Autodesk Inventor part; units mm, degrees
ref_plane "YZ Plane" through (0, 0, 0) normal (1, 0, 0) x (0, 1, 0)
ref_plane "XZ Plane" through (0, 0, 0) normal (0, 1, 0) x (-1, 0, 0)
ref_plane "XY Plane" through (0, 0, 0) normal (0, 0, 1) x (1, 0, 0)
sketch "Sketch1" plane through (0, 0, 0) normal (0, 1, 0) x (-1, 0, 0)
  circle A0 centre (0, 0) radius 2.5
  circle A1 centre (0, 0) radius 3.5
  dimension "d228" = 5
  dimension "d229" = 7
extrude "Extrusion1" add sketch "Sketch1" along normal blind 2
sketch "Sketch2" plane through (0, 2, 0) normal (0, 1, 0) x (1, 0, 0)
  circle A0 centre (0, 0) radius 3.5
  circle A1 centre (0, 0) radius 3.5
  line L0 (-16, -2) -> (0, -3.5)
  circle A2 centre (0, 0) radius 3.5
  line L1 (0, 3.5) -> (-16, 2)
  circle A3 centre (-14, 0) radius 0.75
  arc A4 (-16, 2) -> (-16, -2) centre (-16, 0) ccw
  circle A5 centre (0, 0) radius 1
  circle A6 centre (0, 0) radius 2.5
  circle A7 centre (0, 0) radius 2.5
  dimension "d234" = 1.5
  dimension "d236" = 16
  dimension "d237" = 2
  dimension "d238" = 2
  dimension "d241" = 2
extrude "Extrusion2" add sketch "Sketch2" along normal blind 2 contours A0 L0 L1 | A0 L0 A4 L1
extrude "Extrusion3" add sketch "Sketch2" along normal blind 1 contours A6
extrude "Extrusion4" cut sketch "Sketch2" along normal blind 0.5 contours A6
properties part number "Langbektang houder"
Geometry: final body of the model. Coordinates: model frame, mm. A direction names the side the tool comes from. Coordinates: 2 decimals unless noted, no trailing zeros. Order: outer loops, then holes, each group sorted by start corner. A loop starts at its lowest first (then second) coordinate and runs counter-clockwise, first axis right, second up. Notation, with made-up numbers: (11, 60) - (44, 60) arc R36 cw to (44, 95) - close; hole circle Ø8 at (18, -4). An arc over 180 degrees is marked (long way). Write each question's results on one line, items separated by ' | '.
(1) Section query D-D, the plane y = 0.6. Return the cut outline in (x, z).
Values found:
outline: circle Ø7 at (0, 0); hole circle Ø5 at (0, 0)
(2) Line query: line 1 (X direction, y = 2.9, z = 0); line 2 (X direction, y = 3.4, z = 0); line 3 (Z direction, x = 0, y = 1.45). Output: solid intervals per line, ascending. Write a range as [from, to].
Values found:
line 1: x = [-18, -14.75], [-13.25, -1], [1, 3.5] | line 2: x = [-18, -14.75], [-13.25, -2.5], [2.5, 3.5] | line 3: z = [-3.5, -2.5], [2.5, 3.5]
(3) Section query C-C, the plane x = -14. Return the cut outline in (y, z), plus the area to 3 significant figures.
Values found:
outline: (2, -2.19) - (4, -2.19) - (4, -0.75) - (2, -0.75) - close; (2, 0.75) - (4, 0.75) - (4, 2.19) - (2, 2.19) - close | area: 5.75 mm²
(4) Mould query, pull axis Z, two halves, no side actions, for faces 4 (the face through (-2, 0, -2)), 5 (the face through (-0.165, 1.232, -2.495)), 6 (the face through (-7.89, 2.99, -2.76)). Classes: +Z half, -Z half, draft (parallel to the pull), parting line (faces both ways), or undercut.
Values found:
face 4: draft | face 5: undercut | face 6: -Z half
(5) Set-up query: faces 1 (the face through (3.497, 1.528, -0.154)), 2 (the face through (-14.75, 2.99, 0.03)), 3 (the face through (2.385, 3.493, 0.751)). Return all of +Z, -Z, +X, -X, +Y, -Y with unobstructed straight access to the full face (end or side cutting, diameter ignored); none if empty.
Values found:
face 1: -Y | face 2: +Y, -Y | face 3: +Y
(6) Section query B-B, the plane y = 3.5. Return the cut outline in (x, z).
Values found:
outline: (-16, -2) - (0, -3.5) arc R3.5 ccw to (0, 3.5) - (-16, 2) arc R2 ccw to start; hole circle Ø1.5 at (-14, 0); hole circle Ø5 at (0, 0)
(7) Section query A-A, the plane z = 0. Return the cut outline in (x, y).
Values found:
outline: (-18, 2) - (-14.75, 2) - (-14.75, 4) - (-18, 4) - close; (-13.25, 2) - (-3.5, 2) - (-3.5, 0) - (-2.5, 0) - (-2.5, 2.5) - (-1, 2.5) - (-1, 3) - (-2.5, 3) - (-2.5, 4) - (-13.25, 4) - close; (1, 2.5) - (2.5, 2.5) - (2.5, 0) - (3.5, 0) - (3.5, 4) - (2.5, 4) - (2.5, 3) - (1, 3) - close
(8) First-contact query: pin 1 Ø3 at (x, z) = (0, 0) entering from +Y; pin 2 Ø1.2 at (x, z) = (-14, 0) entering from -Y; pin 3 Ø1 at (x, y) = (-9, 3.5) entering from +Z; pin 4 Ø2 at (x, z) = (-13, 1) entering from -Y. Flat tips, straight axial feed; report the tip coordinate or a pass-through.
Values found:
pin 1: stops at y = 3 | pin 2: passes through | pin 3: stops at z = 2.7 | pin 4: stops at y = 2
